Part model, mm, in its own coordinate system. A direction names the side the tool comes from. Round coordinates to 2 decimals unless told otherwise and drop trailing zeros. Loops run counter-clockwise (first coordinate to the right, second up) from the corner with the lowest first, then second, coordinate; pieces in that order, holes last.
from build123d import *

# Parameters (mm, degrees)
BOSS_EXTRUDE1_DEPTH      = 1.25
BOSS_EXTRUDE1_DEPTH_BACK = 1.25
CUT_EXTRUDE1_DEPTH       = 10.842509843
CUT_EXTRUDE1_DEPTH_BACK  = 10.842509843
BOSS_EXTRUDE4_DEPTH      = 5
BOSS_EXTRUDE4_DEPTH_BACK = 5
BOSS_EXTRUDE2_DEPTH      = 3.75
BOSS_EXTRUDE2_DEPTH_BACK = 6.25
BOSS_EXTRUDE3_DEPTH      = 3.75
BOSS_EXTRUDE3_DEPTH_BACK = 3.75
BOSS_EXTRUDE5_DEPTH      = 0.9375
BOSS_EXTRUDE5_DEPTH_BACK = 2.8125
SKETCH6_W                = 2.5
SKETCH6_H                = 2.5


with BuildPart() as part:
    # Sketch1 → Boss-Extrude1 (new, two sides: drawn at the far end of the back side and taken through both)
    with BuildSketch(Plane.XY.offset(-BOSS_EXTRUDE1_DEPTH_BACK)):
        Polygon((-7.5, -3.75), (-7.5, -6.25), (7.5, -6.25), (7.5, -3.75), (7.5, 3.75), (-7.5, 3.75), align=None)
    extrude(amount=BOSS_EXTRUDE1_DEPTH + BOSS_EXTRUDE1_DEPTH_BACK)

    # Sketch4 → Cut-Extrude1 (cut, two sides: drawn at the far end of the back side and taken through both)
    with BuildSketch(Plane(origin=(0, 0, 0), x_dir=(0, 0, -1), z_dir=(1, 0, 0)).offset(-CUT_EXTRUDE1_DEPTH_BACK)):
        Polygon((-0.816987298, 3.25), (-1.466506351, 3.625), (-1.466506351, 2.875), align=None)
        Polygon((-1.466506351, 1.875), (-0.816987298, 2.25), (-1.466506351, 2.625), align=None)
        Polygon((-1.466506351, 0.875), (-0.816987298, 1.25), (-1.466506351, 1.625), align=None)
        Polygon((-1.466506351, -0.125), (-0.816987298, 0.25), (-1.466506351, 0.625), align=None)
        Polygon((-1.466506351, -1.125), (-0.816987298, -0.75), (-1.466506351, -0.375), align=None)
        Polygon((-1.466506351, -2.125), (-0.816987298, -1.75), (-1.466506351, -1.375), align=None)
        Polygon((-1.466506351, -3.125), (-0.816987298, -2.75), (-1.466506351, -2.375), align=None)
        Polygon((-1.466506351, -4.125), (-0.816987298, -3.75), (-1.466506351, -3.375), align=None)
        Polygon((-1.466506351, -5.125), (-0.816987298, -4.75), (-1.466506351, -4.375), align=None)
        Polygon((-1.466506351, -6.125), (-0.816987298, -5.75), (-1.466506351, -5.375), align=None)
        Polygon((1.466506351, -5.375), (1.466506351, -6.125), (0.816987298, -5.75), align=None)
        Polygon((1.466506351, -4.375), (1.466506351, -5.125), (0.816987298, -4.75), align=None)
        Polygon((1.466506351, -3.375), (1.466506351, -4.125), (0.816987298, -3.75), align=None)
        Polygon((1.466506351, -2.375), (1.466506351, -3.125), (0.816987298, -2.75), align=None)
        Polygon((1.466506351, -1.375), (1.466506351, -2.125), (0.816987298, -1.75), align=None)
        Polygon((1.466506351, -0.375), (1.466506351, -1.125), (0.816987298, -0.75), align=None)
        Polygon((1.466506351, 0.625), (1.466506351, -0.125), (0.816987298, 0.25), align=None)
        Polygon((1.466506351, 1.625), (1.466506351, 0.875), (0.816987298, 1.25), align=None)
        Polygon((1.466506351, 2.625), (1.466506351, 1.875), (0.816987298, 2.25), align=None)
        Polygon((1.466506351, 2.875), (0.816987298, 3.25), (1.466506351, 3.625), align=None)
    extrude(amount=CUT_EXTRUDE1_DEPTH + CUT_EXTRUDE1_DEPTH_BACK, mode=Mode.SUBTRACT)

    # Sketch5 → Boss-Extrude4 (add, two sides: drawn at the far end of the back side and taken through both)
    with BuildSketch(Plane(origin=(0, 0, 0), x_dir=(0, 0, -1), z_dir=(1, 0, 0)).offset(-BOSS_EXTRUDE4_DEPTH_BACK)):
        Polygon((1.683012702, 2.75), (1.033493649, 3.125), (1.033493649, 2.375), align=None)
        Polygon((1.033493649, 1.375), (1.683012702, 1.75), (1.033493649, 2.125), align=None)
        Polygon((1.033493649, 0.375), (1.683012702, 0.75), (1.033493649, 1.125), align=None)
        Polygon((1.033493649, -0.625), (1.683012702, -0.25), (1.033493649, 0.125), align=None)
        Polygon((1.033493649, -1.625), (1.683012702, -1.25), (1.033493649, -0.875), align=None)
        Polygon((1.033493649, -2.625), (1.683012702, -2.25), (1.033493649, -1.875), align=None)
        Polygon((1.033493649, -3.625), (1.683012702, -3.25), (1.033493649, -2.875), align=None)
        Polygon((1.033493649, -4.625), (1.683012702, -4.25), (1.033493649, -3.875), align=None)
        Polygon((1.033493649, -5.625), (1.683012702, -5.25), (1.033493649, -4.875), align=None)
        Polygon((-1.033493649, -4.875), (-1.033493649, -5.625), (-1.683012702, -5.25), align=None)
        Polygon((-1.033493649, -3.875), (-1.033493649, -4.625), (-1.683012702, -4.25), align=None)
        Polygon((-1.033493649, -2.875), (-1.033493649, -3.625), (-1.683012702, -3.25), align=None)
        Polygon((-1.033493649, -1.875), (-1.033493649, -2.625), (-1.683012702, -2.25), align=None)
        Polygon((-1.033493649, -0.875), (-1.033493649, -1.625), (-1.683012702, -1.25), align=None)
        Polygon((-1.033493649, 0.125), (-1.033493649, -0.625), (-1.683012702, -0.25), align=None)
        Polygon((-1.033493649, 1.125), (-1.033493649, 0.375), (-1.683012702, 0.75), align=None)
        Polygon((-1.033493649, 2.125), (-1.033493649, 1.375), (-1.683012702, 1.75), align=None)
        Polygon((-1.033493649, 2.375), (-1.683012702, 2.75), (-1.033493649, 3.125), align=None)
    extrude(amount=BOSS_EXTRUDE4_DEPTH + BOSS_EXTRUDE4_DEPTH_BACK)

    # Sketch2 → Boss-Extrude2 (add, two sides: drawn at the far end of the back side and taken through both)
    with BuildSketch(Plane(origin=(0, 0, 0), x_dir=(1, 0, 0), z_dir=(0, 1, 0)).offset(-BOSS_EXTRUDE2_DEPTH_BACK)):
        Polygon((-7.5, -6.25), (-3.75, -6.25), (-2.5, -3.75), (-5, -3.75), (-5, 3.75), (-2.5, 3.75), (-3.75, 6.25), (-7.5, 6.25), align=None)
        Polygon((7.5, -6.25), (3.75, -6.25), (2.5, -3.75), (5, -3.75), (5, 3.75), (2.5, 3.75), (3.75, 6.25), (7.5, 6.25), align=None)
    extrude(amount=BOSS_EXTRUDE2_DEPTH + BOSS_EXTRUDE2_DEPTH_BACK)

    # Sketch3 → Boss-Extrude3 (add, two sides: drawn at the far end of the back side and taken through both)
    with BuildSketch(Plane.XY.offset(-BOSS_EXTRUDE3_DEPTH_BACK)):
        Polygon((-6.25, -6.25), (-8.75, -6.25), (-10, -3.75), (-6.25, -3.75), align=None)
        Polygon((6.25, -6.25), (8.75, -6.25), (10, -3.75), (6.25, -3.75), align=None)
    extrude(amount=BOSS_EXTRUDE3_DEPTH + BOSS_EXTRUDE3_DEPTH_BACK)

    # Sketch6 → Boss-Extrude5 (add, two sides: drawn at the far end of the back side and taken through both)
    with BuildSketch(Plane(origin=(0, 0, 0), x_dir=(1, 0, 0), z_dir=(0, 1, 0)).offset(-BOSS_EXTRUDE5_DEPTH_BACK)):
        with Locations((-8.75, -5)):
            Rectangle(SKETCH6_W, SKETCH6_H)
        with Locations((-8.75, 5)):
            Rectangle(SKETCH6_W, SKETCH6_H)
        with Locations((8.75, 5)):
            Rectangle(SKETCH6_W, SKETCH6_H)
        with Locations((8.75, -5)):
            Rectangle(SKETCH6_W, SKETCH6_H)
    extrude(amount=BOSS_EXTRUDE5_DEPTH + BOSS_EXTRUDE5_DEPTH_BACK)


solid = part.part
1) Slice it at C-C, the plane y = -1.5. Give the cut face in (x, z).
Values:
outline: (-10, -6.25) - (-3.75, -6.25) - (-2.5, -3.75) - (-5, -3.75) - (-5, -1.25) - (5, -1.25) - (5, -3.75) - (2.5, -3.75) - (3.75, -6.25) - (10, -6.25) - (10, -3.75) - (7.5, -3.75) - (7.5, 3.75) - (10, 3.75) - (10, 6.25) - (3.75, 6.25) - (2.5, 3.75) - (5, 3.75) - (5, 1.25) - (-5, 1.25) - (-5, 3.75) - (-2.5, 3.75) - (-3.75, 6.25) - (-10, 6.25) - (-10, 3.75) - (-7.5, 3.75) - (-7.5, -3.75) - (-10, -3.75) - close
2) Wall check: line 1 along Z through (x, y) = (4.5, -1.5); line 2 along X through (y, z) = (0.75, -2); line 3 along X through (y, z) = (3, -4.25). Give the ranges that are in metal, low to high.
Values:
line 1: z = -6.25 to -3.75, -1.25 to 1.25, 3.75 to 6.25
line 2: x = -7.5 to -5, 5 to 7.5
line 3: x = -7.5 to -2.75, 2.75 to 7.5
3) Tool access for faces 4 (the face through (9, -2.812, -5)), 5 (the face through (-0.07, 2.496, 1.244)), 6 (the face through (-8, -5, -3.75)): list every direction of +Z, -Z, +X, -X, +Y, -Y with a clear straight run to the whole face (end or side of a thin tool).
Values:
face 4: +Z, -Z, +X, -Y
face 5: none
face 6: -Z, -X, -Y
4) Slice it at D-D, the plane z = 2.5. Give the cut face in (x, y).
Values:
outline: (-10, -3.75) - (-8.75, -6.25) - (-5, -6.25) - (-5, 3.75) - (-7.5, 3.75) - (-7.5, -3.75) - close; (5, -6.25) - (8.75, -6.25) - (10, -3.75) - (7.5, -3.75) - (7.5, 3.75) - (5, 3.75) - close
5) Drop flat-ended pins along their axis: pin 1 Ø1.2 at (x, z) = (8.5, -0.5) entering from +Y; pin 2 Ø0.8 at (x, z) = (8, 5) entering from +Y; pin 3 Ø0.8 at (x, y) = (8.5, -5) entering from +Z. Give the stop position or say it passes through.
Values:
pin 1: stops at y = -3.75
pin 2: stops at y = 0.94
pin 3: stops at z = 3.75
6) Mould opens along Z. For faces 1 (the face through (6, -1, 6.25)), 2 (the face through (-0.07, 1.497, 1.244)), 3 (the face through (9, 0.938, -5)) say: released by +Z, released by -Z, zero draft, split by the parting line, or undercut.
Values:
face 1: released by +Z
face 2: undercut
face 3: zero draft
7) Slice it at B-B, the plane z = 4.75. Give the cut face in (x, y).
Values:
outline: (-10, -2.81) - (-7.5, -2.81) - (-7.5, -6.25) - (-3, -6.25) - (-3, 3.75) - (-7.5, 3.75) - (-7.5, 0.94) - (-10, 0.94) - close; (3, -6.25) - (7.5, -6.25) - (7.5, -2.81) - (10, -2.81) - (10, 0.94) - (7.5, 0.94) - (7.5, 3.75) - (3, 3.75) - close
8) Slice it at A-A, the plane x = 7.75. Give the cut face in (y, z), then the cut area to 3 significant figures.
Values:
outline: (-6.25, -3.75) - (-3.75, -3.75) - (-3.75, 3.75) - (-6.25, 3.75) - close; (-2.81, -6.25) - (0.94, -6.25) - (0.94, -3.75) - (-2.81, -3.75) - close; (-2.81, 3.75) - (0.94, 3.75) - (0.94, 6.25) - (-2.81, 6.25) - close
area: 37.5 mm2
